```python
from build123d import *

# Parameters (mm, degrees)
SKETCH207_W     = 104
SKETCH207_H     = 14
SKETCH207_W_2   = 114
SKETCH207_H_2   = 80
SKETCH207_R     = 1.75
SKETCH207_R_2   = 1.25
SKETCH207_W_3   = 24.3
SKETCH207_H_3   = 30
PAD103_DEPTH    = 4
SKETCH208_R     = 1.5
POCKET120_DEPTH = 11


with BuildPart() as part:
    # Sketch207 → Pad103 (new body)
    with BuildSketch(Plane.XY):
        with Locations((57, 7)):
            Rectangle(SKETCH207_W, SKETCH207_H)
        with Locations((57, 54)):
            Rectangle(SKETCH207_W_2, SKETCH207_H_2)
        with Locations((92, 45)):
            Circle(SKETCH207_R, mode=Mode.SUBTRACT)
        with Locations((92, 81.7)):
            Circle(SKETCH207_R, mode=Mode.SUBTRACT)
        with Locations((15, 91.5)):
            Circle(SKETCH207_R_2, mode=Mode.SUBTRACT)
        with Locations((92, 63.5)):
            Rectangle(SKETCH207_W_3, SKETCH207_H_3, mode=Mode.SUBTRACT)
    extrude(amount=PAD103_DEPTH)

    # Sketch208 (on Face2 of Pad103) → Pocket120 (cut)
    with BuildSketch(Plane.XZ.offset(-14)):
        with Locations((2.5, 2)):
            Circle(SKETCH208_R)
        with Locations((111.5, 2)):
            Circle(SKETCH208_R)
    extrude(amount=-POCKET120_DEPTH, mode=Mode.SUBTRACT)


solid = part.part
```
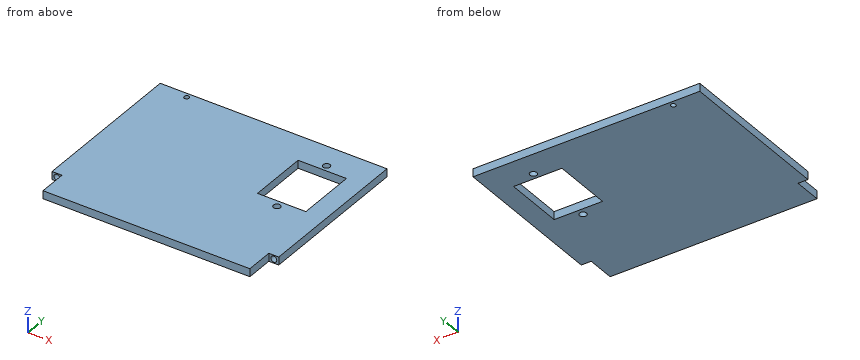
Check sheet for the modelled part. Datum: model origin and axes. Units: mm. Round coordinates to 2 decimals unless told otherwise and drop trailing zeros. Order: outer loops, then holes, each group sorted by start corner. A loop starts at its lowest first (then second) coordinate and runs counter-clockwise, first axis right, second up. Notation, with made-up numbers: (75.25, 57.5) -> (107.25, 57.5) arc R28 ccw to (107.25, 80.5) -> close; hole circle Ø9 at (54.25, -11). An arc over 180 degrees is marked (long way). One line per item, written item: value. Start each with the question number.
Q1. Thickness scan on line 1 (Y direction, x = 92, z = 2.05); line 2 (X direction, y = 18, z = 2.15); line 3 (Y direction, x = 96, z = 2). Record the ranges inside material, lowest first.
Q2. Cross-section at C-C (z = 2.85). Record the boundary of the cut face in (x, y), and give its area (3 significant figures).
Q3. Cross-section at A-A (y = 81.7). Record the boundary of the cut face in (x, z), and give its area (3 significant figures).
Q4. Gauge pin test, flat ends, axial feed: pin 1 Ø1.2 at (y, z) = (67, 2.5) entering from -X; pin 2 Ø2 at (x, y) = (92, 45) entering from +Z; pin 3 Ø1.5 at (x, z) = (2, 2.5) entering from -Y; pin 4 Ø2 at (y, z) = (4, 3) entering from -X. Record the tip position at first contact, or that the pin passes through.
Q5. Cross-section at B-B (x = 15). Record the boundary of the cut face in (y, z), and give its area (3 significant figures).
Q6. Cross-section at D-D (x = 2.5). Record the boundary of the cut face in (y, z), and give its area (3 significant figures).
Completed:
1. line 1: y = 0 to 43.25, 46.75 to 48.5, 78.5 to 79.95, 83.45 to 94
1. line 2: x = 0 to 1.01, 3.99 to 110.01, 112.99 to 114
1. line 3: y = 0 to 48.5, 78.5 to 94
2. outline: (0, 14) -> (1.26, 14) -> (1.26, 25) -> (3.74, 25) -> (3.74, 14) -> (5, 14) -> (5, 0) -> (109, 0) -> (109, 14) -> (110.26, 14) -> (110.26, 25) -> (112.74, 25) -> (112.74, 14) -> (114, 14) -> (114, 94) -> (0, 94) -> close; hole circle Ø2.5 at (15, 91.5); hole (79.85, 48.5) -> (104.15, 48.5) -> (104.15, 78.5) -> (79.85, 78.5) -> close; hole circle Ø3.5 at (92, 45); hole circle Ø3.5 at (92, 81.7)
2. area: 9,770 mm²
3. outline: (0, 0) -> (90.25, 0) -> (90.25, 4) -> (0, 4) -> close; (93.75, 0) -> (114, 0) -> (114, 4) -> (93.75, 4) -> close
3. area: 442 mm²
4. pin 1: stops at x = 0
4. pin 2: passes through
4. pin 3: stops at y = 25
4. pin 4: stops at x = 5
5. outline: (0, 0) -> (90.25, 0) -> (90.25, 4) -> (0, 4) -> close; (92.75, 0) -> (94, 0) -> (94, 4) -> (92.75, 4) -> close
5. area: 366 mm²
6. outline: (14, 0) -> (94, 0) -> (94, 4) -> (14, 4) -> (14, 3.5) -> (25, 3.5) -> (25, 0.5) -> (14, 0.5) -> close
6. area: 287 mm²
